```python
from build123d import *

# Parameters (mm, degrees)
F1_DEPTH = 4
F2_W     = 39.829583
F2_H     = 8
F3_DEPTH = 4
F4_R     = 1.5
F5_DEPTH = 12


with BuildPart() as f1:
    # F0 (on Top) → F1 (new body)
    with BuildSketch(Plane.XY):
        Polygon((-123.954707, -15), (83.954707, -15), (83.954707, -7), (-36.045293, -7), (-36.045293, -4), (123.954707, -4), (123.954707, 4), (-36.045293, 4), (-36.045293, 7), (83.954707, 7), (83.954707, 15), (-123.954707, 15), align=None)
    extrude(amount=F1_DEPTH)

    # F2 (on face) → F3 (join)
    with BuildSketch(Plane.XY.offset(4)):
        with Locations((104.039916, 0)):
            Rectangle(F2_W, F2_H)
    extrude(amount=F3_DEPTH)

    # F4 (on face) → F5 (cut)
    with BuildSketch(Plane.XZ.offset(4)):
        with Locations((108.954707, 4)):
            Circle(F4_R)
    extrude(amount=-F5_DEPTH, mode=Mode.SUBTRACT)


solid = f1.part
```
CAD build for the part. Positions are in the model's coordinates, mm. A direction names the side the tool comes from. Round coordinates to 2 decimals unless told otherwise and drop trailing zeros. Loops run counter-clockwise (first coordinate to the right, second up) from the corner with the lowest first, then second, coordinate; pieces in that order, holes last. Notation, with made-up numbers: (53, -29.75) - (71, -29.75) arc R25 ccw to (71, -9.75) - close; hole circle Ø2 at (80.5, -31). An arc over 180 degrees is marked (long way). Return JSON: item names as keys, results as strings. Group by question number.
Q1. Band-saw the part on A-A on x = -17.5. Give the cut face in (y, z), plus the area to 3 significant figures.
Q2. Band-saw the part on C-C on y = -11.75. Give the cut face in (x, z), plus the area to 3 significant figures.
Q3. Drill centre lines: line 1 along Y through (x, z) = (39.5, 2.75); line 2 along Z through (x, y) = (-16, 0); line 3 along X through (y, z) = (12.5, 3.5). Where is each one in solid material? Low to high. Write a range as [from, to].
Q4. Tool access for faces 5 (the face through (83.955, 11, 2)), 6 (the face through (83.955, -11, 2)), 7 (the face through (25, -7, 2)), 8 (the face through (84.125, 0, 6)): list every direction of +Z, -Z, +X, -X, +Y, -Y with a clear straight run to the whole face (end or side of a thin tool).
Q5. Two-plate mould, pull along Y, no slides. Class faces 1 (the face through (23, 7, 2)), 2 (the face through (123.955, 0, 2)), 3 (the face through (61, -4, 3)), 4 (the face through (-21, -15, 2)): +Y half, -Y half, draft (parallel to the pull), parting line (faces both ways), or undercut.
Q6. Flat gauge pins, fed straight in: pin 1 Ø1.5 at (y, z) = (-6, 3) entering from +X; pin 2 Ø2 at (y, z) = (-9, 2) entering from +X; pin 3 Ø1.2 at (y, z) = (-0.5, 6) entering from -X. Where does each tip first touch, or does it go through?
Q7. Band-saw the part on B-B on x = -47.5. Give the cut face in (y, z), plus the area to 3 significant figures.
Solutions:
{
 "1": {"outline": "(-15, 0) - (-7, 0) - (-7, 4) - (-15, 4) - close; (-4, 0) - (4, 0) - (4, 4) - (-4, 4) - close; (7, 0) - (15, 0) - (15, 4) - (7, 4) - close", "area": "96.0 mm^2"},
 "2": {"outline": "(-123.95, 0) - (83.95, 0) - (83.95, 4) - (-123.95, 4) - close", "area": "832 mm^2"},
 "3": {"line 1": "y = [-15, -7], [-4, 4], [7, 15]", "line 2": "z = [0, 4]", "line 3": "x = [-123.95, 83.95]"},
 "4": {"face 5": "+Z, -Z, +X, +Y", "face 6": "+Z, -Z, +X, -Y", "face 7": "+Z, -Z, +X", "face 8": "+Z, -X, +Y, -Y"},
 "5": {"face 1": "undercut", "face 2": "draft", "face 3": "undercut", "face 4": "-Y half"},
 "6": {"pin 1": "stops at x = -36.05", "pin 2": "stops at x = 83.95", "pin 3": "stops at x = 84.13"},
 "7": {"outline": "(-15, 0) - (15, 0) - (15, 4) - (-15, 4) - close", "area": "120 mm^2"}
}
